Can you work these out from the model? Positions are in its coordinate system, mm. Face numbers are marked on the shaded views. A direction names the side the tool comes from. Give positions to 0.01 mm unless a question says otherwise; leave off trailing zeros. Order: outer loops, then holes, each group sorted by start corner. A loop starts at its lowest first (then second) coordinate and runs counter-clockwise, first axis right, second up. Notation, with made-up numbers: (-15.75, -16) - (9.25, -16) arc R11 ccw to (9.25, -10) - close; hole circle Ø2 at (-6, 84.25). An arc over 180 degrees is marked (long way). Write each question's results on one line, items separated by ' | '. Start each with the question number.
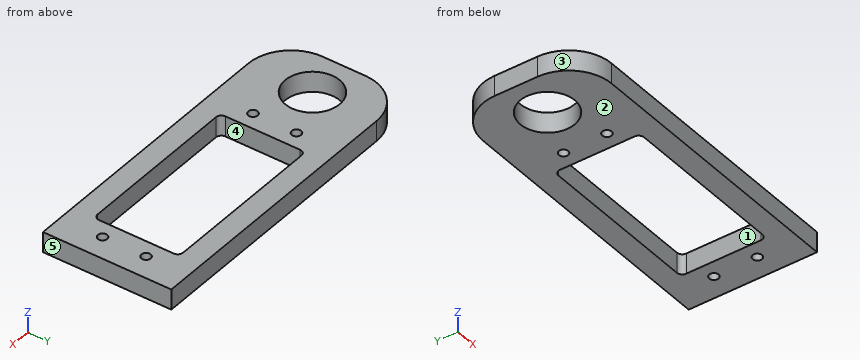
from build123d import *

# Parameters (mm, degrees)
ESQUISSE1_W             = 75
ESQUISSE1_H             = 30
BOSS_EXTRU_1_DEPTH      = 4.7625
CONG_1_R                = 10
ESQUISSE2_R             = 6.35
ENL_V_MAT_EXTRU_1_DEPTH = 6
ENL_V_MAT_EXTRU_2_REACH = 42.669
ESQUISSE3_W             = 40
ESQUISSE3_H             = 20
CONG_2_R                = 1.27
ENL_V_MAT_EXTRU_3_REACH = 42.669
ESQUISSE4_R             = 1.09


with BuildPart() as part:
    # Esquisse1 → Boss.-Extru.1 (new body)
    with BuildSketch(Plane.XY):
        Rectangle(ESQUISSE1_W, ESQUISSE1_H)
    extrude(amount=BOSS_EXTRU_1_DEPTH)

    # Congé1
    cong_1_edges = [part.edges().sort_by_distance(p)[0] for p in [
        (-37.5, -15, 2.38125),
        (-37.5, 15, 2.38125),
    ]]
    fillet(cong_1_edges, radius=CONG_1_R)

    # Esquisse2 → Enlèv. mat.-Extru.1 (cut)
    with BuildSketch(Plane.XY.offset(4.7625)):
        with Locations((-27.5, 0)):
            Circle(ESQUISSE2_R)
    extrude(amount=-ENL_V_MAT_EXTRU_1_DEPTH, mode=Mode.SUBTRACT)

    # Esquisse3 → Enlèv. mat.-Extru.2 (cut, up to next)
    with BuildSketch(Plane.XY.offset(4.7625), mode=Mode.PRIVATE) as enl_v_mat_extru_2_sk1:
        with Locations((8.25, 0)):
            Rectangle(ESQUISSE3_W, ESQUISSE3_H)
    enl_v_mat_extru_2_tool1 = extrude(enl_v_mat_extru_2_sk1.sketch, amount=-ENL_V_MAT_EXTRU_2_REACH, mode=Mode.PRIVATE) & part.part
    add(enl_v_mat_extru_2_tool1.solids().sort_by_distance((8.25, 0, 4.7625))[0], mode=Mode.SUBTRACT)

    # Congé2
    cong_2_edges = [part.edges().sort_by_distance(p)[0] for p in [
        (-11.75, -10, 2.38125),
        (-11.75, 10, 2.38125),
        (28.25, 10, 2.38125),
        (28.25, -10, 2.38125),
    ]]
    fillet(cong_2_edges, radius=CONG_2_R)

    # Esquisse4 → Enlèv. mat.-Extru.3 (cut, up to next)
    with BuildSketch(Plane.XY.offset(4.7625), mode=Mode.PRIVATE) as enl_v_mat_extru_3_sk1:
        with Locations((-15.56, 5.08)):
            Circle(ESQUISSE4_R)
    enl_v_mat_extru_3_tool1 = extrude(enl_v_mat_extru_3_sk1.sketch, amount=-ENL_V_MAT_EXTRU_3_REACH, mode=Mode.PRIVATE) & part.part
    # Esquisse4 → Enlèv. mat.-Extru.3 (cut, up to next)
    with BuildSketch(Plane.XY.offset(4.7625), mode=Mode.PRIVATE) as enl_v_mat_extru_3_sk2:
        with Locations((-15.56, -5.08)):
            Circle(ESQUISSE4_R)
    enl_v_mat_extru_3_tool2 = extrude(enl_v_mat_extru_3_sk2.sketch, amount=-ENL_V_MAT_EXTRU_3_REACH, mode=Mode.PRIVATE) & part.part
    # Esquisse4 → Enlèv. mat.-Extru.3 (cut, up to next)
    with BuildSketch(Plane.XY.offset(4.7625), mode=Mode.PRIVATE) as enl_v_mat_extru_3_sk3:
        with Locations((32.06, -5.08)):
            Circle(ESQUISSE4_R)
    enl_v_mat_extru_3_tool3 = extrude(enl_v_mat_extru_3_sk3.sketch, amount=-ENL_V_MAT_EXTRU_3_REACH, mode=Mode.PRIVATE) & part.part
    # Esquisse4 → Enlèv. mat.-Extru.3 (cut, up to next)
    with BuildSketch(Plane.XY.offset(4.7625), mode=Mode.PRIVATE) as enl_v_mat_extru_3_sk4:
        with Locations((32.06, 5.08)):
            Circle(ESQUISSE4_R)
    enl_v_mat_extru_3_tool4 = extrude(enl_v_mat_extru_3_sk4.sketch, amount=-ENL_V_MAT_EXTRU_3_REACH, mode=Mode.PRIVATE) & part.part
    add(enl_v_mat_extru_3_tool1.solids().sort_by_distance((-15.56, 5.08, 4.7625))[0], mode=Mode.SUBTRACT)
    add(enl_v_mat_extru_3_tool2.solids().sort_by_distance((-15.56, -5.08, 4.7625))[0], mode=Mode.SUBTRACT)
    add(enl_v_mat_extru_3_tool3.solids().sort_by_distance((32.06, -5.08, 4.7625))[0], mode=Mode.SUBTRACT)
    add(enl_v_mat_extru_3_tool4.solids().sort_by_distance((32.06, 5.08, 4.7625))[0], mode=Mode.SUBTRACT)


solid = part.part
Q1. If we section it at B-B (y = 0): Please give me the cut outline in (x, z).
Q2. Which directions (+Z, -Z, +X, -X, +Y, -Y) give clear straight access to the entire face, cutting with the end or side of a thin tool? Please do the marked faces 1 and 2.
Q3. If I drill on probe 1 along Y at (x, z) = (32.06, 1.2); probe 2 along Y at (x, z) = (21.5, 1.15); probe 3 along X at (y, z) = (2.5, 1.5), over which ranges is the centre line in solid material (lowest first)? Write a range as from..to.
Q4. If we section it at D-D (x = -25.5): Please give me the cut outline in (y, z), plus the area to 3 significant figures.
Q5. If we section it at A-A (x = 19): Please give me the cut outline in (y, z), plus the area to 3 significant figures.
Q6. If we section it at C-C (z = 2.75): Please give me the cut outline in (x, y).
Q7. Will these pins go through, and if not, where does the flat tip stop? P1, Ø1.5, axis at x = -14.5, y = -9, coming from the -Z side; P2, Ø1, axis at y = 8.5, z = 3, coming from the -X side.
Q8. Thinking about a two-plate mould opening in X: for the marked faces 3, 4 and 5, which applies, released by +X, released by -X, zero draft, split by the parting line, or undercut?
Findings below:
1) outline: (-37.5, 0) - (-33.85, 0) - (-33.85, 4.76) - (-37.5, 4.76) - close; (-21.15, 0) - (-11.75, 0) - (-11.75, 4.76) - (-21.15, 4.76) - close; (28.25, 0) - (37.5, 0) - (37.5, 4.76) - (28.25, 4.76) - close
2) face 1: +Z, -Z | face 2: -Z, +X, -X, +Y, -Y
3) probe 1: y = -15..-6.17, -3.99..3.99, 6.17..15 | probe 2: y = -15..-10, 10..15 | probe 3: x = -37.5..-33.34, -21.66..-11.75, 28.25..37.5
4) outline: (-15, 0) - (-6.03, 0) - (-6.03, 4.76) - (-15, 4.76) - close; (6.03, 0) - (15, 0) - (15, 4.76) - (6.03, 4.76) - close | area: 85.5 mm2
5) outline: (-15, 0) - (-10, 0) - (-10, 4.76) - (-15, 4.76) - close; (10, 0) - (15, 0) - (15, 4.76) - (10, 4.76) - close | area: 47.6 mm2
6) outline: (-37.5, -5) arc R10 ccw to (-27.5, -15) - (37.5, -15) - (37.5, 15) - (-27.5, 15) arc R10 ccw to (-37.5, 5) - close; hole circle Ø12.7 at (-27.5, 0); hole circle Ø2.18 at (-15.56, -5.08); hole circle Ø2.18 at (-15.56, 5.08); hole (-11.75, -8.73) arc R1.27 ccw to (-10.48, -10) - (26.98, -10) arc R1.27 ccw to (28.25, -8.73) - (28.25, 8.73) arc R1.27 ccw to (26.98, 10) - (-10.48, 10) arc R1.27 ccw to (-11.75, 8.73) - close; hole circle Ø2.18 at (32.06, -5.08); hole circle Ø2.18 at (32.06, 5.08)
7) P1: stops at z = 0 | P2: stops at x = -37.04
8) face 3: released by -X | face 4: undercut | face 5: released by +X
